Source: CAD feature listing. Evaluate the final solid. Frame: model axes, mm. Round coordinates to 2 decimals unless told otherwise and drop trailing zeros. Return JSON: item names as keys, results as strings. Group by question number.
from build123d import *

# Parameters (mm, degrees)
SKETCH1_R           = 12
BOSS_EXTRUDE1_DEPTH = 10
SKETCH2_R           = 7
CUT_EXTRUDE1_DEPTH  = 7
SKETCH3_R           = 4.558249482
CUT_EXTRUDE2_DEPTH  = 2.5


# Read off the part's stored shape, not the designer's step: Cut-Revolve7
with BuildPart() as part:
    # Sketch1 → Boss-Extrude1 (new body)
    with BuildSketch(Plane(origin=(0, 0, 0), x_dir=(1, 0, 0), z_dir=(0, 1, 0))):
        with Locations(Location((0, 0, 0), (0, 0, 270))):
            Circle(SKETCH1_R)
    extrude(amount=BOSS_EXTRUDE1_DEPTH)

    # Sketch2 → Cut-Extrude1 (cut)
    with BuildSketch(Plane.XZ):
        with Locations(Location((0, 0, 0), (0, 0, 270))):
            Circle(SKETCH2_R)
        Polygon((2.95, -1.703183294), (2.95, 1.703183294), (0, 3.406366588), (-2.95, 1.703183294), (-2.95, -1.703183294), (0, -3.406366588), align=None, mode=Mode.SUBTRACT)
    extrude(amount=-CUT_EXTRUDE1_DEPTH, mode=Mode.SUBTRACT)

    # Sketch3 → Cut-Extrude2 (cut)
    with BuildSketch(Plane.XZ):
        Circle(SKETCH3_R)
    extrude(amount=-CUT_EXTRUDE2_DEPTH, mode=Mode.SUBTRACT)

    # Cut-Revolve7 outline → Cut-Revolve7 (revolve, cut)
    with BuildSketch(Plane.XY):
        with BuildLine():
            Line((12, 10), (0.197481425, 10))
            add(Edge.make_bspline(
                [(0.197481425, 10), (8.149812734, 9.330049938), (7.76948814, 8.0260799), (10.078601748, 8.379238452), (8.747465668, 2.511373283), (12, 0)],
                knots=[0, 0, 0, 0, 0, 0, 1, 1, 1, 1, 1, 1], degree=5))
            Line((12, 0), (12, 10))
        make_face()
    revolve(axis=Axis((0, 0, 0), (0, 1, 0)), mode=Mode.SUBTRACT)


solid = part.part
Item 1: Material intervals for probe 1 along X at (y, z) = (4.5, 0); probe 2 along X at (y, z) = (6.5, -0.75); probe 3 along X at (y, z) = (2, 5.25), sorted ascending.
Item 2: Pull-direction query (X, two-part tool) for faces 1 (the flat face through (-5.2, 0, 5.2)), 2 (the flat face through (-1.5, 7, -3)); classes: +X half, -X half, draft (parallel to the pull), parting line (faces both ways), or undercut.
Item 3: First-contact query: pin 1 Ø11 at (x, z) = (0, 0) entering from -Y; pin 2 Ø3 at (x, z) = (-2.5, -7.5) entering from -Y; pin 3 Ø3 at (x, y) = (-1, 5.5) entering from +Z; pin 4 Ø1 at (y, z) = (6, -8.5) entering from -X. Flat tips, straight axial feed; report the tip coordinate or a pass-through.
Here are the results:
{
 "1": {"probe 1": "x = -9.64 to -7, -2.95 to 2.95, 7 to 9.64", "probe 2": "x = -8.96 to -6.96, -2.95 to 2.95, 6.96 to 8.96", "probe 3": "x = -9.1 to -4.63, 4.63 to 9.1"},
 "2": {"face 1": "draft", "face 2": "undercut"},
 "3": {"pin 1": "stops at y = 2.5", "pin 2": "stops at y = 0", "pin 3": "stops at z = 9.75", "pin 4": "stops at x = -4.56"}
}
